For this review, take the finished solid that the model builds, in its own axes (mm). A direction names the side the tool comes from. Round coordinates to 2 decimals unless told otherwise and drop trailing zeros. Order: outer loops, then holes, each group sorted by start corner. A loop starts at its lowest first (then second) coordinate and runs counter-clockwise, first axis right, second up. Notation, with made-up numbers: (16, 15.5) - (63, 15.5) arc R31 cw to (63, 43.5) - close; hole circle Ø8 at (25.5, -9.75). An arc over 180 degrees is marked (long way). One line per question, with ' | ' between items.
```python
from build123d import *

# Parameters (mm, degrees)
SKETCH_1_W      = 25
SKETCH_1_H      = 280
EXTRUDE_1_DEPTH = 147.5
SKETCH_2_W      = 80
SKETCH_2_H      = 25
EXTRUDE_2_DEPTH = 280
EXTRUDE_3_DEPTH = 25


with BuildPart() as part:
    # 草图1 → 凸台-拉伸1 (new, symmetric)
    with BuildSketch(Plane.XY):
        Rectangle(SKETCH_1_W, SKETCH_1_H)
    extrude(amount=EXTRUDE_1_DEPTH, both=True)

    # 草图2 → 凸台-拉伸2 (add)
    with BuildSketch(Plane(origin=(0, 140, 0), x_dir=(1, 0, 0), z_dir=(0, 1, 0))):
        with Locations((52.5, -135)):
            Rectangle(SKETCH_2_W, SKETCH_2_H)
    extrude(amount=-EXTRUDE_2_DEPTH)

    # 草图4 → 凸台-拉伸3 (add)
    with BuildSketch(Plane(origin=(0, 130, 0), x_dir=(1, 0, 0), z_dir=(0, 1, 0))):
        Polygon((12.5, 127.5), (32.5, 127.5), (92.5, -102.5), (92.5, -122.5), (12.5, -122.5), align=None)
    extrude_3 = extrude(amount=-EXTRUDE_3_DEPTH)

    # 镜向1: 凸台-拉伸3 across plane
    add(extrude_3.mirror(Plane.ZX))


solid = part.part
```
(1) We need section A-A on x = 85. State the section outline as (y, z) points, plus the area to 3 significant figures.
Output values:
outline: (-140, 122.5) - (-130, 122.5) - (-130, 73.75) - (-105, 73.75) - (-105, 122.5) - (105, 122.5) - (105, 73.75) - (130, 73.75) - (130, 122.5) - (140, 122.5) - (140, 147.5) - (-140, 147.5) - close | area: 9,440 mm^2
(2) Mouldability with a two-part tool opening along Y and no side actions: class faces 1 (the flat face through (44, 105, 24)), 2 (the flat face through (22, 118, -127.5)), 3 (the flat face through (44, 130, 24)), 4 (the flat face through (9, -140, 32)) as released by +Y, released by -Y, zero draft, split by the parting line, or undercut.
Output values:
face 1: undercut | face 2: zero draft | face 3: released by +Y | face 4: released by -Y
(3) Insertion check: pin 1 (24 mm diameter, centred on x = 63, z = -21, fed in from +Y); pin 2 (24 mm diameter, centred on x = 71, z = 21.5, fed in from -Y); pin 3 (24 mm diameter, centred on x = 62.5, y = -38, fed in from -Z). Each pin has a flat end and moves straight along its axis. Give the tip position at first contact, or say it passes through.
Output values:
pin 1: y = 130 | pin 2: y = -130 | pin 3: z = 122.5
(4) We need section C-C on z = -117.5. State the section outline as (x, y) points, plus the area to 3 significant figures.
Output values:
outline: (-12.5, -140) - (12.5, -140) - (12.5, -130) - (35.11, -130) - (35.11, -105) - (12.5, -105) - (12.5, 105) - (35.11, 105) - (35.11, 130) - (12.5, 130) - (12.5, 140) - (-12.5, 140) - close | area: 8,130 mm^2
(5) We need section B-B on y = 117. State the section outline as (x, z) points.
Output values:
outline: (-12.5, -147.5) - (12.5, -147.5) - (12.5, -127.5) - (32.5, -127.5) - (92.5, 102.5) - (92.5, 147.5) - (-12.5, 147.5) - close
(6) For faces 5 (the flat face through (52, 1, 122.5)), 6 (the flat face through (52, 135, 122.5)), 7 (the flat face through (9, 140, 32)), 8 (the flat face through (44, -130, 24)), 9 (the flat face through (22, -118, -127.5)), list the 3-axis set-ups (+Z, -Z, +X, -X, +Y, -Y) from which the entire face can be reached by the end or side of a thin tool; tool diameter is ignored.
Output values:
face 5: -Z, +X | face 6: -Z, +X, +Y | face 7: +Z, -Z, +X, -X, +Y | face 8: -Z, +X, -Y | face 9: -Z, +X, +Y, -Y
(7) We need section D-D on y = -44.5. State the section outline as (x, z) points.
Output values:
outline: (-12.5, -147.5) - (12.5, -147.5) - (12.5, 122.5) - (92.5, 122.5) - (92.5, 147.5) - (-12.5, 147.5) - close
(8) For probe 1 along Y at (x, z) = (69.5, 25.5); probe 2 along X at (y, z) = (-49, 47.5); probe 3 along Z at (x, y) = (36.5, -73), list the stretches that pass through material, from the lowest coordinate up. Write a range as [from, to].
Output values:
probe 1: [-130, -105], [105, 130] | probe 2: [-12.5, 12.5] | probe 3: [122.5, 147.5]
